from build123d import *

# Parameters (mm, degrees)
SKETCH1_W           = 36
SKETCH1_H           = 12.5
BOSS_EXTRUDE1_DEPTH = 1.5
SKETCH2_R           = 0.5
CUT_EXTRUDE1_DEPTH  = 20.113149924
LPATTERN1_COUNT     = 4
LPATTERN1_PITCH     = 2.54
SKETCH3_W           = 7.5
SKETCH3_H           = 12
BOSS_EXTRUDE2_DEPTH = 5.8
SKETCH4_W           = 1.5
SKETCH4_H           = 2
CUT_EXTRUDE2_DEPTH  = 23.532254659
CHAMFER1_SIZE       = 1.5
SKETCH5_W           = 30
SKETCH5_H           = 11.5
BOSS_EXTRUDE3_DEPTH = 1.6
EXTRUDE_THIN1_START = -0.8
EXTRUDE_THIN1_DEPTH = 7.5
SKETCH7_W           = 26
SKETCH7_H           = 9.2
CUT_EXTRUDE3_DEPTH  = 0.1


with BuildPart() as part:
    # Sketch1 → Boss-Extrude1 (new body)
    with BuildSketch(Plane(origin=(0, 0, 0), x_dir=(1, 0, 0), z_dir=(0, 1, 0))):
        Rectangle(SKETCH1_W, SKETCH1_H)
    extrude(amount=BOSS_EXTRUDE1_DEPTH)

    # Sketch2 → Cut-Extrude1 (cut, through all)
    with BuildSketch(Plane(origin=(0, 1.5, 0), x_dir=(1, 0, 0), z_dir=(0, 1, 0))):
        with Locations(Location((-16.73, -3.81, 0), (0, 0, 270))):
            Circle(SKETCH2_R)
    cut_extrude1 = extrude(amount=-CUT_EXTRUDE1_DEPTH, mode=Mode.SUBTRACT)

    # LPattern1: Cut-Extrude1 ×4
    with Locations(*[(0, 0, -i * LPATTERN1_PITCH) for i in range(1, LPATTERN1_COUNT)]):
        add(cut_extrude1, mode=Mode.SUBTRACT)

    # Sketch3 → Boss-Extrude2 (add)
    with BuildSketch(Plane.XZ):
        with Locations((14, 0)):
            Rectangle(SKETCH3_W, SKETCH3_H)
    extrude(amount=BOSS_EXTRUDE2_DEPTH)

    # Sketch4 → Cut-Extrude2 (cut, through all)
    with BuildSketch(Plane.XY.offset(6)):
        with Locations((11, -4.8)):
            Rectangle(SKETCH4_W, SKETCH4_H)
    extrude(amount=-CUT_EXTRUDE2_DEPTH, mode=Mode.SUBTRACT)

    # Chamfer1
    chamfer1_edges = [part.edges().sort_by_distance(p)[0] for p in [
        (10.25, -3.8, 0),
    ]]
    chamfer(chamfer1_edges, length=CHAMFER1_SIZE - 0.0001)  # a hair under: the kernel refuses the full size

    # Sketch5 → Boss-Extrude3 (add)
    with BuildSketch(Plane(origin=(0, 1.5, 0), x_dir=(1, 0, 0), z_dir=(0, 1, 0))):
        with Locations((0.5, 0)):
            Rectangle(SKETCH5_W, SKETCH5_H)
    extrude(amount=BOSS_EXTRUDE3_DEPTH)

    # Sketch6 → Extrude-Thin1 (add)
    with BuildSketch(Plane.XY.offset(5.75).offset(EXTRUDE_THIN1_START)):
        with BuildLine():
            Line((15.5, 1.5), (16.75, 1.5))
            ThreePointArc((16.75, 1.5), (17.2, 1.95), (16.75, 2.4))
            Line((16.75, 2.4), (15.5, 2.4))
            Line((15.5, 2.4), (15.5, 2.3))
            Line((15.5, 2.3), (16.75, 2.3))
            ThreePointArc((16.75, 2.3), (17.1, 1.95), (16.75, 1.6))
            Line((16.75, 1.6), (15.5, 1.6))
            Line((15.5, 1.6), (15.5, 1.5))
        make_face()
    extrude(amount=-EXTRUDE_THIN1_DEPTH)

    # Sketch7 → Cut-Extrude3 (cut)
    with BuildSketch(Plane(origin=(0, 3.1, 0), x_dir=(1, 0, 0), z_dir=(0, 1, 0))):
        with Locations((-1.4, 1.05)):
            Rectangle(SKETCH7_W, SKETCH7_H)
    extrude(amount=-CUT_EXTRUDE3_DEPTH, mode=Mode.SUBTRACT)


solid = part.part
Model file for the job. Use its own axes, mm. A direction names the side the tool comes from. Round coordinates to 2 decimals unless told otherwise and drop trailing zeros. Loops run counter-clockwise (first coordinate to the right, second up) from the corner with the lowest first, then second, coordinate; pieces in that order, holes last. Notation, with made-up numbers: (22, 49) -> (66, 49) arc R31 cw to (66, 83) -> close; hole circle Ø7 at (11.25, -19). An arc over 180 degrees is marked (long way). Answer as CSV lines item,"result". Start each with the question number.
1) Tool access for faces 5 (the face through (-2, 3, -1)), 6 (the face through (18, 1, 0)), 7 (the face through (10.25, -1, 0)), 8 (the face through (0, 2, 5.75)), 9 (the face through (17.75, -3, 0)): list every direction of +Z, -Z, +X, -X, +Y, -Y with a clear straight run to the whole face (end or side of a thin tool).
2) Mould opens along Z. For faces 1 (the face through (-16.392, 0.76, 3.441)), 2 (the face through (0, 1, 6.25)), 3 (the face through (0, 2, -5.75)), 4 (the face through (-18, 1, 0)) say: +Z half, -Z half, draft (parallel to the pull), parting line (faces both ways), or undercut.
3) Probe line 1 along X through (y, z) = (0.55, 3.81); line 2 along Y through (x, z) = (-2.5, 3.75); line 3 along Y through (x, z) = (9, -0.75). List the from-to ranges inside material, lowest first.
4) Slice it at B-B (x = -16.73). List the corners of the cut face in (y, z), plus the area to 4 significant figures.
5) Slice it at D-D (y = -5). List the corners of the cut face in (x, z).
6) Slice it at A-A (z = 1.27). State how many separate pieces and enclosed holes the cut face has, plus the area to 3 significant figures.
7) Pin check, flat tips, straight feed: P1, Ø1.7, axis at y = -2, z = 0, coming from the +X side; P2, Ø1.8, axis at y = -1, z = 1, coming from the -X side; P3, Ø0.5, axis at x = 8, y = 2.5, coming from the -Z side. Stop position of each tip, or through.
8) Slice it at C-C (x = -4.5). List the corners of the cut face in (y, z), plus the area to 3 significant figures.
Filled in:
1,face 5,"+Y"
1,face 6,"+Z, -Z, +X, +Y, -Y"
1,face 7,"+Z, -Z, -X, -Y"
1,face 8,"+Z, +X, -X, +Y"
1,face 9,"+Z, -Z, +X, -Y"
2,face 1,"undercut"
2,face 2,"+Z half"
2,face 3,"-Z half"
2,face 4,"draft"
3,line 1,"x = -18 to -17.23, -16.23 to 18"
3,line 2,"y = 0 to 3.1"
3,line 3,"y = 0 to 3"
4,outline,"(0, -6.25) -> (1.5, -6.25) -> (1.5, -4.31) -> (0, -4.31) -> close; (0, -3.31) -> (1.5, -3.31) -> (1.5, -1.77) -> (0, -1.77) -> close; (0, -0.77) -> (1.5, -0.77) -> (1.5, 0.77) -> (0, 0.77) -> close; (0, 1.77) -> (1.5, 1.77) -> (1.5, 3.31) -> (0, 3.31) -> close; (0, 4.31) -> (1.5, 4.31) -> (1.5, 6.25) -> (0, 6.25) -> close"
4,area,"12.75 mm2"
5,outline,"(11.75, -6) -> (17.75, -6) -> (17.75, 6) -> (11.75, 6) -> close"
6,separate pieces,"2"
6,enclosed holes,"1"
6,area,"138 mm2"
7,P1,"stops at x = 17.75"
7,P2,"stops at x = 10.25"
7,P3,"stops at z = -5.75"
8,outline,"(0, -6.25) -> (1.5, -6.25) -> (1.5, -5.75) -> (3.1, -5.75) -> (3.1, -5.65) -> (3, -5.65) -> (3, 3.55) -> (3.1, 3.55) -> (3.1, 5.75) -> (1.5, 5.75) -> (1.5, 6.25) -> (0, 6.25) -> close"
8,area,"36.2 mm2"
